from build123d import *

# Parameters (mm, degrees)
F0_W     = 200
F0_H     = 50
F1_DEPTH = 15
F3_DEPTH = 15
F4_R     = 3
F5_DEPTH = 15.001
F6_R     = 3


with BuildPart() as f1:
    # F0 (on Top) → F1 (new body)
    with BuildSketch(Plane.XY):
        Rectangle(F0_W, F0_H)
    extrude(amount=F1_DEPTH)

    # F2 (on face) → F3 (join)
    with BuildSketch(Plane.XZ.offset(25)):
        with BuildLine():
            Line((25, 15), (20, 15))
            ThreePointArc((20, 15), (0, 5), (-20, 15))
            Line((-20, 15), (-25, 15))
            Line((-25, 15), (-25, 0))
            Line((-25, 0), (25, 0))
            Line((25, 0), (25, 15))
        make_face()
        with BuildLine():
            ThreePointArc((-20, 15), (-23.7170824513, 22.0943058496), (-25, 30))
            Line((-25, 30), (-25, 15))
            Line((-25, 15), (-20, 15))
        make_face()
        with BuildLine():
            Line((25, 15), (25, 30))
            ThreePointArc((25, 30), (23.7170824513, 22.0943058496), (20, 15))
            Line((20, 15), (25, 15))
        make_face()
        with BuildLine():
            ThreePointArc((-20, 15), (0, 5), (20, 15))
            Line((20, 15), (-20, 15))
        make_face()
        with BuildLine():
            ThreePointArc((20, 15), (23.7170824513, 22.0943058496), (25, 30))
            Line((25, 30), (10, 30))
            ThreePointArc((10, 30), (0, 20), (-10, 30))
            Line((-10, 30), (-25, 30))
            ThreePointArc((-25, 30), (-23.7170824513, 22.0943058496), (-20, 15))
            Line((-20, 15), (20, 15))
        make_face()
        with BuildLine():
            Line((10, 30), (25, 30))
            ThreePointArc((25, 30), (0, 55), (-25, 30))
            Line((-25, 30), (-10, 30))
            ThreePointArc((-10, 30), (0, 40), (10, 30))
        make_face()
    extrude(amount=-F3_DEPTH)

    # F4 (on face) → F5 (cut, through all)
    with BuildSketch(Plane.XY.offset(15)):
        with Locations((-85, 10)):
            Circle(F4_R)
        with Locations((-85, -10)):
            Circle(F4_R)
        with Locations((85, 10)):
            Circle(F4_R)
        with Locations((85, -10)):
            Circle(F4_R)
    extrude(amount=-F5_DEPTH, mode=Mode.SUBTRACT)

    # F6
    f6_edges = [f1.edges().sort_by_distance(p)[0] for p in [
        (-62.5, -25, 15),
        (-100, 0, 15),
        (0, 25, 15),
        (100, 0, 15),
        (62.5, -25, 15),
        (25, -17.5, 15),
        (-25, -17.5, 15),
        (-25, -10, 22.5),
        (0, -25, 0),
        (100, 0, 0),
        (0, 25, 0),
        (-100, 0, 0),
        (-25, -25, 22.5),
        (0, -25, 55),
        (25, -25, 22.5),
        (0, -10, 15),
        (0, -10, 55),
        (25, -10, 22.5),
    ]]
    fillet(f6_edges, radius=F6_R)


solid = f1.part
Design review of the part built by this model. Coordinates are the model's own, in mm. A direction names the side the tool comes from. Coordinates: 2 decimals unless noted, no trailing zeros. Order: outer loops, then holes, each group sorted by start corner. A loop starts at its lowest first (then second) coordinate and runs counter-clockwise, first axis right, second up. Notation, with made-up numbers: M 69.5,74.25 L 81.5,74.25 A16 ccw 81.5,97.25 Z; hole C -26,52 d3. An arc over 180 degrees is marked long. Use a Markdown table: item, result.
(1) For faces 1 (the flat face through (-25, -18, 24)), 2 (the flat face through (-5, -10, 39)), 3 (the flat face through (25, -18, 24)), list the 3-axis set-ups (+Z, -Z, +X, -X, +Y, -Y) from which the entire face can be reached by the end or side of a thin tool; tool diameter is ignored.
Worked answers:
| item | result |
|---|---|
| face 1 | +Z, -X, +Y, -Y |
| face 2 | +Z, +X, -X, +Y |
| face 3 | +Z, +X, +Y, -Y |
(2) Add section A-A (x = 0). Give the boundary of the cut face in (y, z).
Worked answers:
| item | result |
|---|---|
| outline | M -25,3 A3 ccw -22,0 L 22,0 A3 ccw 25,3 L 25,12 A3 ccw 22,15 L -7,15 A3 cw -10,18 L -10,20 L -25,20 Z; M -25,40 L -10,40 L -10,52 A3 ccw -13,55 L -22,55 A3 ccw -25,52 Z |
(3) Add section D-D (y = 10). Give the boundary of the cut face in (x, z).
Worked answers:
| item | result |
|---|---|
| outline | M -100,3 A3 ccw -97,0 L -88,0 L -88,15 L -97,15 A3 ccw -100,12 Z; M -82,0 L 82,0 L 82,15 L -82,15 Z; M 88,0 L 97,0 A3 ccw 100,3 L 100,12 A3 ccw 97,15 L 88,15 Z |
(4) Add section C-C (x = 85). Give the boundary of the cut face in (y, z).
Worked answers:
| item | result |
|---|---|
| outline | M -25,3 A3 ccw -22,0 L -13,0 L -13,15 L -22,15 A3 ccw -25,12 Z; M -7,0 L 7,0 L 7,15 L -7,15 Z; M 13,0 L 22,0 A3 ccw 25,3 L 25,12 A3 ccw 22,15 L 13,15 Z |
(5) Draft analysis for pull direction X (two halves, no side actions). For faces 4 (the cylindrical face through (82, -10, 8)), 5 (the cylindrical face through (-88, 10, 8)), 6 (the cylindrical face through (0.55, -17.563, 54.994)), 7 (the flat face through (100, 0, 7)), state which applies: released by +X, released by -X, zero draft, split by the parting line, or undercut.
Worked answers:
| item | result |
|---|---|
| face 4 | undercut |
| face 5 | undercut |
| face 6 | split by the parting line |
| face 7 | released by +X |
(6) Wall thickness on probe 1 along Y at (x, z) = (85, 8); probe 2 along Z at (x, y) = (-36.5, -21); probe 3 along X at (y, z) = (-7.5, 13): over which ranges is each line inside the solid? List them lowest first.
Worked answers:
| item | result |
|---|---|
| probe 1 | y = -25 to -13, -7 to 7, 13 to 25 |
| probe 2 | z = 0 to 15 |
| probe 3 | x = -99.83 to -86.66, -83.34 to 83.34, 86.66 to 99.83 |
(7) Add section B-B (y = 18). Give the boundary of the cut face in (x, z).
Worked answers:
| item | result |
|---|---|
| outline | M -100,3 A3 ccw -97,0 L 97,0 A3 ccw 100,3 L 100,12 A3 ccw 97,15 L -97,15 A3 ccw -100,12 Z |
(8) For P1, Ø17, axis at x = -6.5, z = 37.5, coming from the +Y side; P2, Ø4.5, axis at y = -16.5, z = 26, coming from the +X side; P3, Ø4, axis at x = -10, y = 15, coming from the +Z side; P4, Ø12, axis at x = 78, y = 5.5, coming from the -Z side, all flat-tipped, find the tip position at first contact; note any pin that passes through.
Worked answers:
| item | result |
|---|---|
| P1 | stops at y = -10 |
| P2 | stops at x = 25 |
| P3 | stops at z = 15 |
| P4 | stops at z = 0 |
